Verification items for the finished model (mm, model axes). A direction names the side the tool comes from. Coordinates: 2 decimals unless noted, no trailing zeros. Order: outer loops, then holes, each group sorted by start corner. A loop starts at its lowest first (then second) coordinate and runs counter-clockwise, first axis right, second up. Notation, with made-up numbers: M -35.5,69 L -5.5,69 A18 cw -5.5,81 Z; hole C 69,-18 d2. An arc over 180 degrees is marked long. Return JSON: item names as keys, results as strings.
Autodesk Inventor part; units mm, degrees
ref_plane "YZ Plane" through (0, 0, 0) normal (1, 0, 0) x (0, 1, 0)
ref_plane "XZ Plane" through (0, 0, 0) normal (0, 1, 0) x (-1, 0, 0)
ref_plane "XY Plane" through (0, 0, 0) normal (0, 0, 1) x (1, 0, 0)
sketch "Sketch1" plane through (0, 0, 0) normal (0, 0, 1) x (1, 0, 0)
  line L0 (0, 20) -> (20, 20)
  line L1 (20, 20) -> (20, 0)
  line L2 (20, 0) -> (0, 0)
  line L3 (0, 0) -> (0, 20)
  circle A0 centre (10, 10) radius 2.5
  dimension "d0" = 20
  dimension "d1" = 20
  dimension "d5" = 10
  dimension "d6" = 10
  dimension "d7" = 5
extrude "Extrusion2" add sketch "Sketch1" along normal blind 5
sketch "Sketch3" plane through (0, 0, 0) normal (0, 0, -1) x (-1, 0, 0)
  line L0 (-20, 20) -> (0, 20)
  line L1 (0, 20) -> (0, 0)
  line L2 (-20, 20) -> (0, 20)
  line L3 (0, 20) -> (0, 0)
  line L4 (0, 0) -> (-20, 0)
  line L5 (-20, 0) -> (-20, 20)
  circle A0 centre (-10, 10) radius 4.5
  dimension "d10" = 9
extrude "Extrusion3" add sketch "Sketch3" along normal blind 6
equation "\"d1\" = d0"
properties part number "Touchscreen mount v04 screw test"
Q1. Tool access check on faces 1 (the face through (10, 0, -1)), 2 (the face through (12, 8, 0)). Record the directions out of +Z, -Z, +X, -X, +Y, -Y that give a thin tool (end or side, any length) a straight path to the whole face; none if there is none.
Values:
{"face 1": "+Z, -Z, +X, -X, -Y", "face 2": "-Z"}
Q2. Cross-section at A-A, the plane x = 10. Record the boundary of the cut face in (y, z), and give its area (3 significant figures).
Values:
{"outline": "M 0,-6 L 5.5,-6 L 5.5,0 L 7.5,0 L 7.5,5 L 0,5 Z; M 12.5,0 L 14.5,0 L 14.5,-6 L 20,-6 L 20,5 L 12.5,5 Z", "area": "141 mm^2"}
Q3. Cross-section at D-D, the plane y = 13.5. Record the boundary of the cut face in (x, z).
Values:
{"outline": "M 0,-6 L 7.17,-6 L 7.17,0 L 12.83,0 L 12.83,-6 L 20,-6 L 20,5 L 0,5 Z"}
Q4. Material ranges on line 1 along Y through (x, z) = (10, -3.3); line 2 along Y through (x, z) = (10, 2.4); line 3 along Z through (x, y) = (12, 11.75), recorded low to high.
Values:
{"line 1": "0 to 5.5, 14.5 to 20", "line 2": "0 to 7.5, 12.5 to 20", "line 3": "0 to 5"}
Q5. Cross-section at C-C, the plane z = -0.5. Record the boundary of the cut face in (x, y), and give its area (3 significant figures).
Values:
{"outline": "M 0,0 L 20,0 L 20,20 L 0,20 Z; hole C 10,10 d9", "area": "336 mm^2"}
Q6. Go/stop test with a flat-tipped pin: pin 1 (4.5 mm diameter, centred on x = 10.5, y = 9, fed in from -Z). Record where the tip stops, or that it passes through.
Values:
{"pin 1": "z = 0"}
Q7. Draft check along X on faces 3 (the face through (0, 10, -1)), 4 (the face through (10, 15, -6)), 5 (the face through (5.708, 8.648, -2.958)). Enter one of: pulls with the +X half, pulls with the -X half, needs draft (parallel to the pull), parting line crosses it, or undercut.
Values:
{"face 3": "pulls with the -X half", "face 4": "needs draft", "face 5": "undercut"}
